Verification items for the finished model (mm, model axes). Face numbers are marked on the shaded views. A direction names the side the tool comes from. Round coordinates to 2 decimals unless told otherwise and drop trailing zeros. Write each loop counter-clockwise with the first axis right and the second up, starting at its lowest first coordinate (ties: lowest second). Pieces come first, ordered by that corner, then holes.
from build123d import *

# Parameters (mm, degrees)
F0_R      = 32
F1_DEPTH  = 20
F2_R      = 17.5
F3_DEPTH  = 3
F5_DEPTH  = 5
F6_R      = 32
F6_R_2    = 10
F7_DEPTH  = 8
F8_R      = 5.5
F9_DEPTH  = 17.001
F10_R     = 2
F11_DEPTH = 20.001


with BuildPart() as f1:
    # F0 (on Front) → F1 (new body)
    with BuildSketch(Plane.XZ):
        Circle(F0_R)
    extrude(amount=-F1_DEPTH)

    # F2 (on Front) → F3 (cut)
    with BuildSketch(Plane.XZ):
        Circle(F2_R)
    extrude(amount=-F3_DEPTH, mode=Mode.SUBTRACT)

    # F4 (on face) → F5 (cut)
    with BuildSketch(Plane.XZ):
        with BuildLine():
            Line((32, 3.5), (14, 3.5))
            ThreePointArc((14, 3.5), (10.5, 0), (14, -3.5))
            Line((14, -3.5), (32, -3.5))
            Line((32, -3.5), (32, 3.5))
        make_face()
        with BuildLine():
            ThreePointArc((-14, -3.5), (-10.5, 0), (-14, 3.5))
            Line((-14, 3.5), (-32, 3.5))
            Line((-32, 3.5), (-32, -3.5))
            Line((-32, -3.5), (-14, -3.5))
        make_face()
    extrude(amount=-F5_DEPTH, mode=Mode.SUBTRACT)

    # F6 (on face) → F7 (cut)
    with BuildSketch(Plane(origin=(0, 20, 0), x_dir=(-1, 0, 0), z_dir=(0, 1, 0))):
        Circle(F6_R)
        Circle(F6_R_2, mode=Mode.SUBTRACT)
    extrude(amount=-F7_DEPTH, mode=Mode.SUBTRACT)

    # F8 (on face) → F9 (cut, through all)
    with BuildSketch(Plane.XZ.offset(-3)):
        Circle(F8_R)
    extrude(amount=-F9_DEPTH, mode=Mode.SUBTRACT)

    # F10 (on Front) → F11 (cut, through all)
    with BuildSketch(Plane.XZ):
        with Locations((-22.5, 0)):
            Circle(F10_R)
        with Locations((22.5, 0)):
            Circle(F10_R)
    extrude(amount=-F11_DEPTH, mode=Mode.SUBTRACT)


solid = f1.part
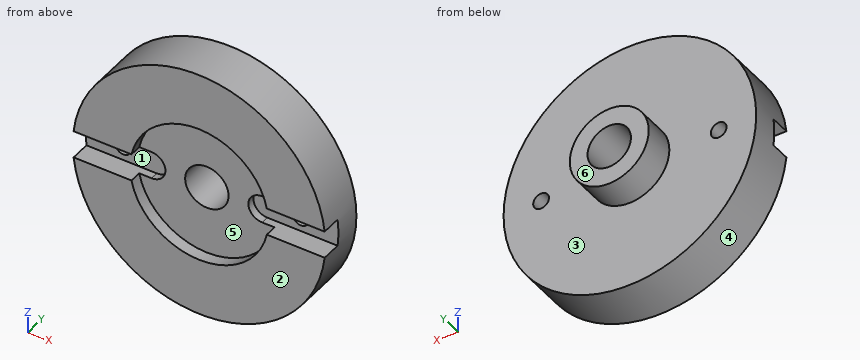
Q1. Sectioned sample at D-D (x = -26.5). Enter the section's corners in (y, z).
Recorded:
outline: (0, -17.94) - (12, -17.94) - (12, 17.94) - (0, 17.94) - (0, 3.5) - (5, 3.5) - (5, -3.5) - (0, -3.5) - close
Q2. Material ranges on line 1 along Y through (x, z) = (8, 0.5); line 2 along Y through (x, z) = (-21.5, -9.5); line 3 along Z through (x, y) = (-9.5, 1.75), recorded low to high.
Recorded:
line 1: y = 3 to 20
line 2: y = 0 to 12
line 3: z = -30.56 to -14.7, 14.7 to 30.56
Q3. Sectioned sample at A-A (z = 0). Enter the section's corners in (x, y).
Recorded:
outline: (-32, 5) - (-24.5, 5) - (-24.5, 12) - (-32, 12) - close; (-20.5, 5) - (-10.5, 5) - (-10.5, 3) - (-5.5, 3) - (-5.5, 20) - (-10, 20) - (-10, 12) - (-20.5, 12) - close; (5.5, 3) - (10.5, 3) - (10.5, 5) - (20.5, 5) - (20.5, 12) - (10, 12) - (10, 20) - (5.5, 20) - close; (24.5, 5) - (32, 5) - (32, 12) - (24.5, 12) - close
Q4. Tool access check on the marked faces 1, 2 and 3. Record the directions out of +Z, -Z, +X, -X, +Y, -Y that give a thin tool (end or side, any length) a straight path to the whole face; none if there is none.
Recorded:
face 1: -X, -Y
face 2: +Z, -Z, +X, -X, -Y
face 3: +Y
Q5. Sectioned sample at C-C (y = 9.25). Enter the section's corners in (x, z).
Recorded:
outline: circle Ø64 at (0, 0); hole circle Ø4 at (-22.5, 0); hole circle Ø11 at (0, 0); hole circle Ø4 at (22.5, 0)
Q6. Sectioned sample at B-B (x = 0). Enter the section's corners in (y, z).
Recorded:
outline: (0, -32) - (12, -32) - (12, -10) - (20, -10) - (20, -5.5) - (3, -5.5) - (3, -17.5) - (0, -17.5) - close; (0, 17.5) - (3, 17.5) - (3, 5.5) - (20, 5.5) - (20, 10) - (12, 10) - (12, 32) - (0, 32) - close
Q7. Depth check by flat-ended pin: P1, Ø6, axis at x = -23, y = 13.5, coming from the +Z side; P2, Ø2.5, axis at x = -24.5, y = 3.5, coming from the -Z side; P3, Ø4, axis at x = -0.5, y = 2, coming from the -Z side; P4, Ø5, axis at x = 2, y = 16, coming from the -Z side. Enter the tip coordinate at first touch or a pass-through.
Recorded:
P1: stops at z = 24.65
P2: stops at z = -21.99
P3: stops at z = -32
P4: stops at z = -10
Q8. Release check for a two-part mould opening along Z. For the marked faces 4, 5 and 6 record: released by +Z, released by -Z, zero draft, split by the parting line, or undercut.
Recorded:
face 4: split by the parting line
face 5: undercut
face 6: zero draft
